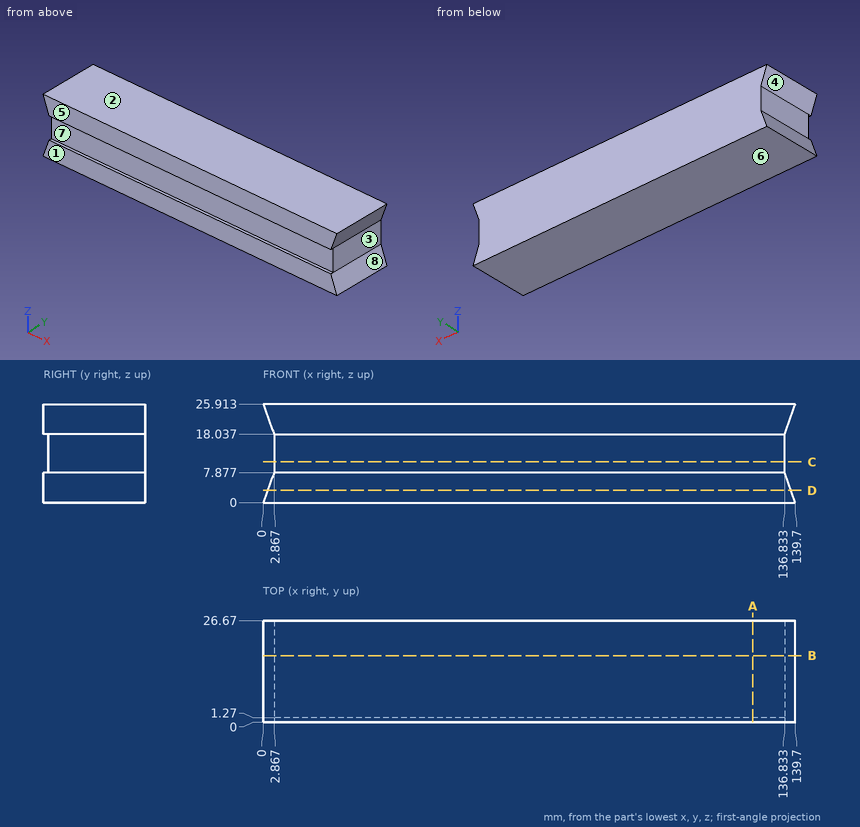
Can you work these out from the drawing? Everything is in mm from the part's minimum corner. A direction names the side the tool comes from. Coordinates: 2 decimals unless noted, no trailing zeros. Loops run counter-clockwise (first coordinate to the right, second up) from the corner with the lowest first, then second, coordinate; pieces in that order, holes last. Notation, with made-up numbers: (52.5, 7) - (58.5, 7) arc R11 cw to (58.5, 19) - close; hole circle Ø9 at (83, -12.75). An arc over 180 degrees is marked (long way). Answer as CSV lines item,"result".
Q1. We'd pull the mould along Z, two halves only. Please class the marked faces 1, 2 and 3: pulls with the +Z half, pulls with the -Z half, needs draft (parallel to the pull), parting line crosses it, or undercut.
Response:
face 1,"needs draft"
face 2,"pulls with the +Z half"
face 3,"undercut"
Q2. If we section it at B-B, the plane y = 17.5: Write out the boundary of the cut face in (x, z).
Response:
outline,"(0, 0) - (139.7, 0) - (136.83, 7.88) - (136.83, 18.04) - (139.7, 25.91) - (0, 25.91) - (2.87, 18.04) - (2.87, 7.88) - close"
Q3. If we section it at D-D, the plane z = 3.25: Write out the boundary of the cut face in (x, y).
Response:
outline,"(1.18, 0) - (138.52, 0) - (138.52, 26.67) - (1.18, 26.67) - close"
Q4. If we section it at A-A, the plane x = 128.5: Write out the boundary of the cut face in (y, z), and give its area (3 significant figures).
Response:
outline,"(0, 0) - (26.67, 0) - (26.67, 25.91) - (0, 25.91) - (0, 18.04) - (1.27, 18.04) - (1.27, 7.88) - (0, 7.88) - close"
area,"678 mm2"
Q5. For pin 1 (1.5 mm diameter, centred on y = 22.5, z = 9, fed in from -X); pin 2 (5 mm diameter, centred on y = 6.5, z = 7.5, fed in from -X); pin 3 (5 mm diameter, centred on y = 20.5, z = 19, fed in from +X); pin 4 (10 mm diameter, centred on x = 101.5, z = 21, fed in from -Y), each with a flat end and sliding along its axis, tell me the tip position at first contact or that it passes through.
Response:
pin 1,"x = 2.87"
pin 2,"x = 1.82"
pin 3,"x = 138.09"
pin 4,"y = 0"
Q6. If we section it at C-C, the plane z = 10.75: Write out the boundary of the cut face in (x, y), and give its area (3 significant figures).
Response:
outline,"(2.87, 1.27) - (136.83, 1.27) - (136.83, 26.67) - (2.87, 26.67) - close"
area,"3,400 mm2"
Q7. If I drill on L1, parallel to X at y = 21.25, z = 15; L2, parallel to Y at x = 54.5, z = 9; L3, parallel to X at y = 21.5, z = 4 (1 decimal), over which ranges is the centre line in solid material (lowest first)? Write a range as [from, to].
Response:
L1,"[2.87, 136.83]"
L2,"[1.27, 26.67]"
L3,"[1.5, 138.2]"
Q8. For the marked faces 4, 5, 6, 7 and 8, which set-ups out of +Z, -Z, +X, -X, +Y, -Y let a thin tool reach every point of the face, with its end or its side?
Response:
face 4,"-X, +Y, -Y"
face 5,"+Z, -Z, +X, -X, -Y"
face 6,"-Z, +X, -X, +Y, -Y"
face 7,"+X, -X, -Y"
face 8,"+X, +Y, -Y"
